Study the drawing (mm; zero at the part's minimum x, y, z) and answer. A direction names the side the tool comes from. Coordinates: 2 decimals unless noted, no trailing zeros. Loops run counter-clockwise (first coordinate to the right, second up) from the corner with the lowest first, then second, coordinate; pieces in that order, holes last. Notation, with made-up numbers: (-14.75, 84.25) - (41.25, 84.25) arc R11 ccw to (41.25, 88.25) - close; hole circle Ø1 at (1, -32). An arc over 180 degrees is marked (long way). Use CSV: the item, a comma, the result in double quotes.
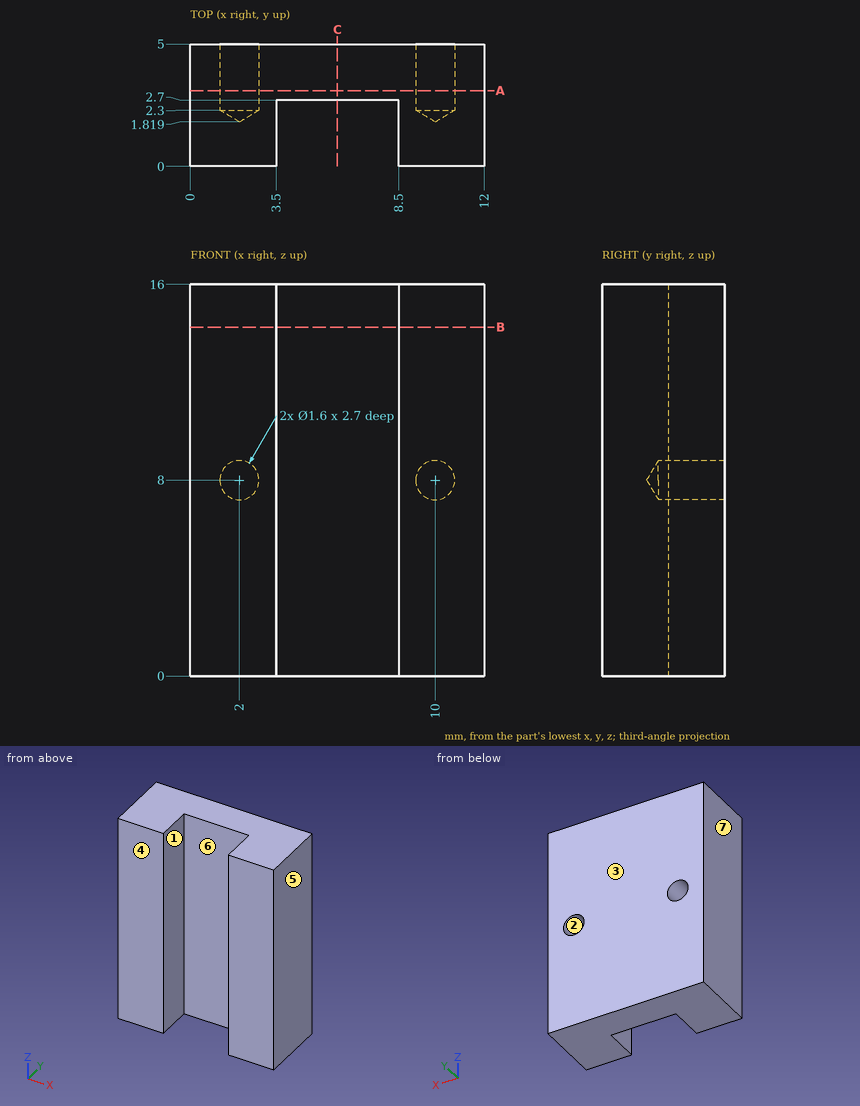
Q1. The part is cut by section B-B on z = 14.25. Determine the outline of the cut face in (x, y), and give its area (3 significant figures).
Reported:
outline,"(0, 0) - (3.5, 0) - (3.5, 2.7) - (8.5, 2.7) - (8.5, 0) - (12, 0) - (12, 5) - (0, 5) - close"
area,"46.5 mm²"
Q2. Find the intervals of material crossed by probe 1 along X at (y, z) = (4.15, 8); probe 2 along X at (y, z) = (1.8, 8.25); probe 3 along Z at (x, y) = (2, 3.7), in increasing order. Write a range as [from, to].
Reported:
probe 1,"x = [0, 1.2], [2.8, 9.2], [10.8, 12]"
probe 2,"x = [0, 3.5], [8.5, 12]"
probe 3,"z = [0, 7.2], [8.8, 16]"
Q3. A tool of negligible diameter and unlimited length cuts with its end or side. For the marked faces 1, 2 and 3, from which of +Z, -Z, +X, -X, +Y, -Y can it reach the whole face along a straight path? Write none if from no direction.
Reported:
face 1,"+Z, -Z, -Y"
face 2,"+Y"
face 3,"+Z, -Z, +X, -X, +Y"
Q4. The part is cut by section A-A on y = 3.1. Determine the outline of the cut face in (x, z).
Reported:
outline,"(0, 0) - (12, 0) - (12, 16) - (0, 16) - close; hole circle Ø1.6 at (2, 8); hole circle Ø1.6 at (10, 8)"
Q5. Given P1, Ø1.5, axis at x = 7, z = 3.5, coming from the -Y side, flat-ended and moving along its own axis, determine where the tip first touches the part or whether it passes through.
Reported:
P1,"stops at y = 2.7"
Q6. The part is cut by section C-C on x = 6. Determine the outline of the cut face in (y, z).
Reported:
outline,"(2.7, 0) - (5, 0) - (5, 16) - (2.7, 16) - close"
Q7. For a pull along X with two mould halves and no side action, classify the marked faces 4, 5, 6 and 7 as +X half, -X half, draft (parallel to the pull), parting line (faces both ways), or undercut.
Reported:
face 4,"draft"
face 5,"+X half"
face 6,"undercut"
face 7,"-X half"
